from build123d import *

# Parameters (mm, degrees)
SKETCH2_R                       = 6.35
BOSS_EXTRUDE1_DEPTH             = 30.9499
TAP_DRILL_FOR_1_4_20_TAP1_D     = 5.1054
TAP_DRILL_FOR_1_4_20_TAP1_DEPTH = 12.7
TAP_DRILL_FOR_1_4_20_TAP1_TIP   = 1.533816902
SKETCH6_R                       = 3.175
BOSS_EXTRUDE2_DEPTH             = 6.35
CUT_EXTRUDE1_DEPTH              = 39.365707865
CUT_EXTRUDE1_DEPTH_BACK         = 39.365707865
SKETCH7_W                       = 1.5875
SKETCH7_H                       = 9.525


with BuildPart() as part:
    # Sketch2 → Boss-Extrude1 (new body)
    with BuildSketch(Plane(origin=(0, 0, 0), x_dir=(0, 1, 0), z_dir=(0, 0, 1))):
        with Locations(Location((0, 0, 0), (0, 0, 270))):
            Circle(SKETCH2_R)
    extrude(amount=BOSS_EXTRUDE1_DEPTH)

    # Tap Drill for 1/4-20 Tap1
    with Locations(Plane(origin=(0, 0, 0), x_dir=(-1, 0, 0), z_dir=(0, 0, -1))):
        with Locations((0, 0)):
            Hole(TAP_DRILL_FOR_1_4_20_TAP1_D / 2, depth=TAP_DRILL_FOR_1_4_20_TAP1_DEPTH)
            with Locations((0, 0, -(TAP_DRILL_FOR_1_4_20_TAP1_DEPTH + TAP_DRILL_FOR_1_4_20_TAP1_TIP / 2))):  # 118° drill point
                Cone(0, TAP_DRILL_FOR_1_4_20_TAP1_D / 2, TAP_DRILL_FOR_1_4_20_TAP1_TIP, mode=Mode.SUBTRACT)

    # Sketch6 → Boss-Extrude2 (add)
    with BuildSketch(Plane.XY.offset(30.9499)):
        Circle(SKETCH6_R)
    extrude(amount=BOSS_EXTRUDE2_DEPTH)

    # Sketch7 → Cut-Extrude1 (cut, two sides: drawn at the far end of the back side and taken through both)
    with BuildSketch(Plane.YZ.offset(-CUT_EXTRUDE1_DEPTH_BACK)):
        with Locations((-5.55625, 16.6624)):
            Rectangle(SKETCH7_W, SKETCH7_H)
        with Locations((5.55625, 16.6624)):
            Rectangle(SKETCH7_W, SKETCH7_H)
    extrude(amount=CUT_EXTRUDE1_DEPTH + CUT_EXTRUDE1_DEPTH_BACK, mode=Mode.SUBTRACT)


solid = part.part
Input: part model. Units: mm. Frame: model coordinates. A direction names the side the tool comes from. Round coordinates to 2 decimals unless told otherwise and drop trailing zeros. Write each loop counter-clockwise with the first axis right and the second up, starting at its lowest first coordinate (ties: lowest second). Pieces come first, ordered by that corner, then holes.
1) Cut plane D-D (z = 26.5). Return the cut outline in (x, y).
2) Contact query for flat-ended pins moving along their axis: P1, Ø1, axis at y = 3.5, z = 15.5, coming from the -X side; P2, Ø1.5, axis at x = 1.5, z = 23.5, coming from the +Y side; P3, Ø2.5, axis at x = -1, z = 15, coming from the -Y side. Output: stop coordinate, or through.
3) Reachability of faces 4 (the flat face through (0, 0, 37.3)), 5 (the cylindrical face through (2.435, 0.767, 6.439)), 6 (the flat face through (0, 5, 21.425)), 7 (the flat face through (0, -5, 11.9)), 8 (the cylindrical face through (-0.69, -3.1, 34.08)) from +Z, -Z, +X, -X, +Y, -Y: full face, straight path, thin tool, end or side. Return the list, or none.
4) Cut plane B-B (z = 16.5). Return the cut outline in (x, y).
5) Cut plane A-A (z = 6). Return the cut outline in (x, y).
6) Cut plane C-C (x = -3.75). Return the cut outline in (y, z).
7) Ray query, L1, parallel to Y at x = 0, z = 9.5; L2, parallel to Z at x = -1.75, y = -5.5; L3, parallel to Z at x = 3, y = -3.75. Return the intervals inside material, ascending.
8) Draft query along Z for faces 1 (the flat face through (0, -5, 21.425)), 2 (the flat face through (3, 0, 0)), 3 (the flat face through (-2, 3, 30.95)). Return one class per face: pulls with the +Z half, pulls with the -Z half, needs draft (parallel to the pull), parting line crosses it, or undercut.
Geometry says:
1. outline: circle Ø12.7 at (0, 0)
2. P1: stops at x = -5.6
2. P2: stops at y = 6.31
2. P3: stops at y = -4.76
3. face 4: +Z, +X, -X, +Y, -Y
3. face 5: -Z
3. face 6: +X, -X, +Y
3. face 7: +X, -X, -Y
3. face 8: +Z
4. outline: (-4.2, -4.76) - (4.2, -4.76) arc R6.35 ccw to (4.2, 4.76) - (-4.2, 4.76) arc R6.35 ccw to start
5. outline: circle Ø12.7 at (0, 0); hole circle Ø5.11 at (0, 0)
6. outline: (-5.12, 0) - (5.12, 0) - (5.12, 11.9) - (4.76, 11.9) - (4.76, 21.42) - (5.12, 21.42) - (5.12, 30.95) - (-5.12, 30.95) - (-5.12, 21.42) - (-4.76, 21.42) - (-4.76, 11.9) - (-5.12, 11.9) - close
7. L1: y = -6.35 to -2.55, 2.55 to 6.35
7. L2: z = 0 to 11.9, 21.42 to 30.95
7. L3: z = 0 to 30.95
8. face 1: undercut
8. face 2: pulls with the -Z half
8. face 3: pulls with the +Z half
